Could you check a few things on this model? Use its own coordinates, in mm. Face numbers are marked on the shaded views. A direction names the side the tool comes from. Coordinates: 2 decimals unless noted, no trailing zeros. Loops run counter-clockwise (first coordinate to the right, second up) from the corner with the lowest first, then second, coordinate; pieces in that order, holes last.
1) Thinking about a two-plate mould opening in X: for the marked faces 1, 2, 3 and 4, which applies, released by +X, released by -X, zero draft, split by the parting line, or undercut?
2) Imagine slicing it at B-B on x = -15.5. Please give me the cut outline in (y, z), plus the area to 3 significant figures.
3) Imagine slicing it at C-C on y = 26. Please give me the cut outline in (x, z).
4) If I drill on line 1 along X through (y, z) = (34.5, 3.2); line 2 along Y through (x, z) = (0, 2.95); line 3 along Y through (x, z) = (-15.5, 1.55), over which ranges is the centre line in solid material (lowest first)?
5) Imagine slicing it at A-A on x = 0. Please give me the cut outline in (y, z), plus the area to 3 significant figures.
6) Imagine slicing it at D-D on z = 1.25. Please give me the cut outline in (x, y).
7) For the marked faces 5 and 6, which set-ups out of +Z, -Z, +X, -X, +Y, -Y let a thin tool reach every point of the face, with its end or its side?
8) Will these pins go through, and if not, where does the flat tip stop? P1, Ø8, axis at x = 6.5, y = 30, coming from the -Z side; P2, Ø2, axis at x = -7, z = 2, coming from the -Y side; P3, Ø2, axis at y = 40, z = 3, coming from the +X side.
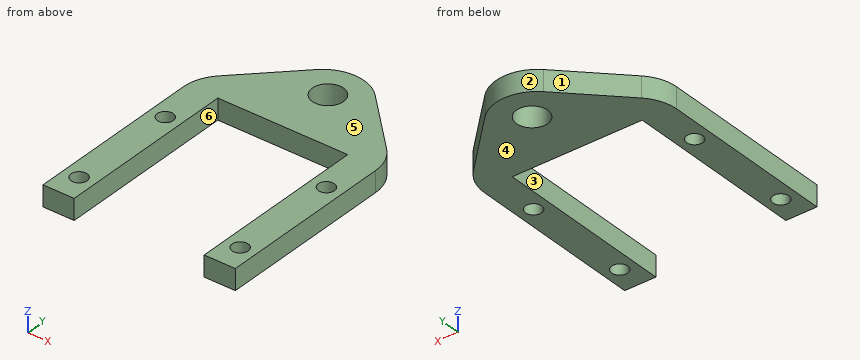
```python
from build123d import *

# Parameters (mm, degrees)
SKETCH_1_R      = 3
SKETCH_1_R_2    = 1.55
EXTRUDE_1_DEPTH = 4
FILLET_1_R      = 8


with BuildPart() as part:
    # 草图1 → 凸台-拉伸1 (new body)
    with BuildSketch(Plane.XY):
        Polygon((-12.5, 0), (-18.5, 0), (-18.5, 37.5), (0, 56), (18.5, 37.5), (18.5, 0), (12.5, 0), (12.5, 35), (-12.5, 35), align=None)
        with Locations((0, 46)):
            Circle(SKETCH_1_R, mode=Mode.SUBTRACT)
        with Locations((-15.5, 5)):
            Circle(SKETCH_1_R_2, mode=Mode.SUBTRACT)
        with Locations((-15.5, 26)):
            Circle(SKETCH_1_R_2, mode=Mode.SUBTRACT)
        with Locations(Location((15.5, 5, 0), (0, 0, 180))):
            Circle(SKETCH_1_R_2, mode=Mode.SUBTRACT)
        with Locations(Location((15.5, 26, 0), (0, 0, 180))):
            Circle(SKETCH_1_R_2, mode=Mode.SUBTRACT)
    extrude(amount=EXTRUDE_1_DEPTH)

    # 圆角1
    fillet_1_edges = [part.edges().sort_by_distance(p)[0] for p in [
        (-18.5, 37.5, 2),
        (0, 56, 2),
        (18.5, 37.5, 2),
    ]]
    fillet(fillet_1_edges, radius=FILLET_1_R)


solid = part.part
```
Filled in:
1. face 1: released by -X
1. face 2: split by the parting line
1. face 3: undercut
1. face 4: zero draft
2. outline: (0, 0) - (3.45, 0) - (3.45, 4) - (0, 4) - close; (6.55, 0) - (24.45, 0) - (24.45, 4) - (6.55, 4) - close; (27.55, 0) - (40.5, 0) - (40.5, 4) - (27.55, 4) - close
2. area: 137 mm2
3. outline: (-18.5, 0) - (-17.05, 0) - (-17.05, 4) - (-18.5, 4) - close; (-13.95, 0) - (-12.5, 0) - (-12.5, 4) - (-13.95, 4) - close; (12.5, 0) - (13.95, 0) - (13.95, 4) - (12.5, 4) - close; (17.05, 0) - (18.5, 0) - (18.5, 4) - (17.05, 4) - close
4. line 1: x = -18.49 to -12.5, 12.5 to 18.49
4. line 2: y = 35 to 43, 49 to 52.69
4. line 3: y = 0 to 3.45, 6.55 to 24.45, 27.55 to 40.5
5. outline: (35, 0) - (43, 0) - (43, 4) - (35, 4) - close; (49, 0) - (52.69, 0) - (52.69, 4) - (49, 4) - close
5. area: 46.7 mm2
6. outline: (-18.5, 0) - (-12.5, 0) - (-12.5, 35) - (12.5, 35) - (12.5, 0) - (18.5, 0) - (18.5, 34.19) arc R8 ccw to (16.16, 39.84) - (5.66, 50.34) arc R8 ccw to (-5.66, 50.34) - (-16.16, 39.84) arc R8 ccw to (-18.5, 34.19) - close; hole circle Ø3.1 at (-15.5, 5); hole circle Ø3.1 at (-15.5, 26); hole circle Ø6 at (0, 46); hole circle Ø3.1 at (15.5, 5); hole circle Ø3.1 at (15.5, 26)
7. face 5: +Z, +X, -X, +Y, -Y
7. face 6: +Z, -Z, -Y
8. P1: passes through
8. P2: stops at y = 35
8. P3: stops at x = 16.89
